Work out the finished part from the listing and answer in its coordinate system (mm). A direction names the side the tool comes from. Give positions to 0.01 mm unless a question says otherwise; leave off trailing zeros. Write each loop counter-clockwise with the first axis right and the second up, starting at its lowest first coordinate (ties: lowest second). Pieces come first, ordered by that corner, then holes.
1) Determine the mould class of faces 6 (the face through (0, 1.25, 1)), 7 (the face through (-19, -28.75, 1)), 8 (the face through (71, -8, 1)), 9 (the face through (-62, -28, 1)) for opening direction X: pulls with the +X half, pulls with the -X half, needs draft (parallel to the pull), parting line crosses it, or undercut.
2) Find section D-D (x = -49.5). Determine the outline of the cut face in (y, z).
3) A tool of negligible diameter and unlimited length cuts with its end or side. For faces 1 (the face through (19, 1.25, 1)), 2 (the face through (43, -27, 1)), 3 (the face through (-72, -10.625, 1)), 4 (the face through (-67, 26.25, 1)), 5 (the face through (67, -26.25, 1)), from which of +Z, -Z, +X, -X, +Y, -Y can it reach the whole face along a straight path? Write none if from no direction.
4) Find section A-A (x = -17). Determine the outline of the cut face in (y, z), plus the area to 4 significant figures.
5) Straight lines are drawn through the part: probe 1 along Y at (x, z) = (-38, 2.45); probe 2 along X at (y, z) = (7, 0.75); probe 3 along Y at (x, z) = (-24.5, 2.2). For each, find the intervals that lie inside material, in ascending order.
6) Find section C-C (y = 8.5). Determine the outline of the cut face in (x, z), plus the area to 3 significant figures.
7) Find section B-B (z = 1.85). Count the separate pieces of the cut face and the enclosed holes in it, plus the area to 3 significant figures.
8) Given pin 1 Ø0.8 at (x, z) = (72, 1) entering from -Y (3 decimals); pin 2 Ø0.8 at (x, z) = (30, 2) entering from -Y; pin 3 Ø0.8 at (y, z) = (27.5, 1) entering from -X, each flat-ended and moving along its own axis, determine where each tip first touches the part or whether it passes through.
```python
from build123d import *

# Parameters (mm, degrees)
SKETCH1_W           = 10
SKETCH1_H           = 2.5
BOSS_EXTRUDE1_DEPTH = 2.5


with BuildPart() as part:
    # Sketch1 → Boss-Extrude1 (new body)
    with BuildSketch(Plane.XY):
        Polygon((-62, 26.25), (-62, 28.75), (-52, 28.75), (-52, 26.25), (-43, 26.25), (-43, 28.75), (-33, 28.75), (-33, 26.25), (-24, 26.25), (-24, 28.75), (-14, 28.75), (-14, 26.25), (-5, 26.25), (-5, 28.75), (5, 28.75), (5, 26.25), (14, 26.25), (14, 28.75), (24, 28.75), (24, 26.25), (33, 26.25), (33, 28.75), (43, 28.75), (43, 26.25), (52, 26.25), (52, 28.75), (62, 28.75), (62, 26.25), (71, 26.25), (71, 20.625), (73.5, 20.625), (73.5, 10.625), (71, 10.625), (71, 5), (73.5, 5), (73.5, -5), (71, -5), (71, -10.625), (73.5, -10.625), (73.5, -20.625), (71, -20.625), (71, -26.25), (62, -26.25), (62, -28.75), (52, -28.75), (52, -26.25), (43, -26.25), (43, -28.75), (33, -28.75), (33, -26.25), (24, -26.25), (24, -28.75), (14, -28.75), (14, -26.25), (5, -26.25), (5, -28.75), (-5, -28.75), (-5, -26.25), (-14, -26.25), (-14, -28.75), (-24, -28.75), (-24, -26.25), (-33, -26.25), (-33, -28.75), (-43, -28.75), (-43, -26.25), (-52, -26.25), (-52, -28.75), (-62, -28.75), (-62, -26.25), (-71, -26.25), (-71, -20.625), (-73.5, -20.625), (-73.5, -10.625), (-71, -10.625), (-71, -5), (-73.5, -5), (-73.5, 5), (-71, 5), (-71, 10.625), (-73.5, 10.625), (-73.5, 20.625), (-71, 20.625), (-71, 26.25), align=None)
        with Locations((-38, 0)):
            Rectangle(SKETCH1_W, SKETCH1_H, mode=Mode.SUBTRACT)
        with Locations((-57, 0)):
            Rectangle(SKETCH1_W, SKETCH1_H, mode=Mode.SUBTRACT)
        with Locations((-19, 0)):
            Rectangle(SKETCH1_W, SKETCH1_H, mode=Mode.SUBTRACT)
        Rectangle(SKETCH1_W, SKETCH1_H, mode=Mode.SUBTRACT)
        with Locations((19, 0)):
            Rectangle(SKETCH1_W, SKETCH1_H, mode=Mode.SUBTRACT)
        with Locations((38, 0)):
            Rectangle(SKETCH1_W, SKETCH1_H, mode=Mode.SUBTRACT)
        with Locations((57, 0)):
            Rectangle(SKETCH1_W, SKETCH1_H, mode=Mode.SUBTRACT)
    extrude(amount=BOSS_EXTRUDE1_DEPTH)


solid = part.part
```
Results:
1. face 6: undercut
1. face 7: needs draft
1. face 8: pulls with the +X half
1. face 9: pulls with the -X half
2. outline: (-26.25, 0) - (26.25, 0) - (26.25, 2.5) - (-26.25, 2.5) - close
3. face 1: +Z, -Z
3. face 2: +Z, -Z, -Y
3. face 3: +Z, -Z, -X
3. face 4: +Z, -Z, -X, +Y
3. face 5: +Z, -Z, +X, -Y
4. outline: (-28.75, 0) - (-1.25, 0) - (-1.25, 2.5) - (-28.75, 2.5) - close; (1.25, 0) - (28.75, 0) - (28.75, 2.5) - (1.25, 2.5) - close
4. area: 137.5 mm2
5. probe 1: y = -28.75 to -1.25, 1.25 to 28.75
5. probe 2: x = -71 to 71
5. probe 3: y = -26.25 to 26.25
6. outline: (-71, 0) - (71, 0) - (71, 2.5) - (-71, 2.5) - close
6. area: 355 mm2
7. separate pieces: 1
7. enclosed holes: 7
7. area: 7,780 mm2
8. pin 1: stops at y = -20.625
8. pin 2: stops at y = -26.25
8. pin 3: stops at x = -62
